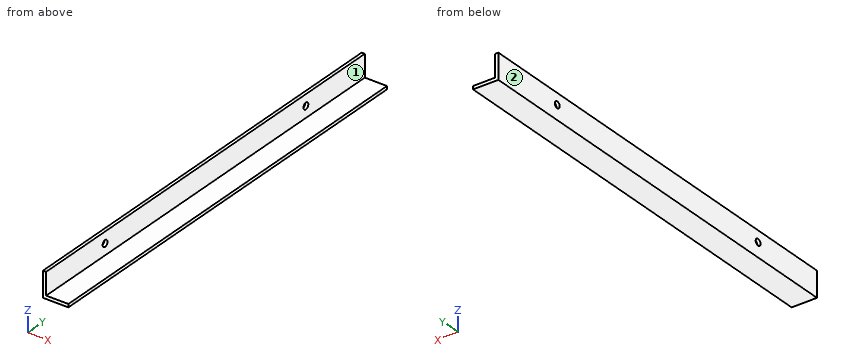
Autodesk Fusion 360 part; units mm, degrees
sketch "Sketch1" plane through (0, 0, 0) normal (0, 1, 0) x (1, 0, 0)
  line L0 (0, -25.4) -> (0, 0)
  line L1 (0, 0) -> (25.4, 0)
  line L2 (12.7, -12.7) -> (11.05, -11.05) construction
  line L3 (3.175, -25.4) -> (3.175, -3.175)
  line L4 (3.175, -3.175) -> (25.4, -3.175)
  line L5 (25.4, -3.175) -> (25.4, 0)
  line L6 (0, -25.4) -> (3.175, -25.4)
  dimension "d1" = 25.4
  dimension "d2" = 25.4
  dimension "d13" = 3.175
extrude "Extrude1" add sketch "Sketch1" along normal blind 215
hole "Hole3" at (3.175, 135.512, 14.2875) direction (-1, 0, 0) diameter 6.5 end through all
mirror "Mirror1" about plane through (0, 0, 0) normal (0, 1, 0) of bodies 1 merged
equation "d5 = ( 430 / 2 ) * 1 mm"
equation "d27 = ( 22.225 / 2 ) * 1 mm"
The model under review builds one solid part; all positions refer to its coordinate system, in mm. Face numbers are marked on the shaded views. A direction names the side the tool comes from. Round coordinates to 2 decimals unless told otherwise and drop trailing zeros. Write each loop counter-clockwise with the first axis right and the second up, starting at its lowest first coordinate (ties: lowest second). Pieces come first, ordered by that corner, then holes. Notation, with made-up numbers: M 10.25,80 L 57.25,80 A17 ccw 57.25,113 Z; hole C -21,41.5 d8. An arc over 180 degrees is marked long. Use CSV: the item, a comma, the result in double quotes. Start each with the question number.
(1) Tool access review of the marked faces 1 and 2: name each direction out of +Z, -Z, +X, -X, +Y, -Y from which nothing blocks a thin tool from reaching the whole face with its end or side.
(2) We need section A-A, the plane y = -1.5. State the section outline as (x, z) points (3 decimals), then the cut area to 3 significant figures.
(3) We need section B-B, the plane x = 7. State the section outline as (y, z) points (3 decimals), then the cut area to 3 significant figures.
(4) Clearance check with flat-ended pins moving along their axes: P1, Ø5, axis at y = -135.51, z = 14.29, coming from the -X side; P2, Ø6, axis at x = 7.5, y = 4.5, coming from the +Z side (3 decimals); P3, Ø8, axis at y = 9, z = 13, coming from the +X side (3 decimals). State where each tip first meets the part, or that it passes through.
(5) For line 1 along Z through (x, y) = (9.5, -92) (3 decimals), list the stretches that pass through material, from the lowest coordinate up.
(6) We need section C-C, the plane z = 21. State the section outline as (x, y) points (3 decimals), then the cut area to 3 significant figures.
Findings:
1,face 1,"+Z, +X, +Y, -Y"
1,face 2,"+Z, -Z, -X, +Y, -Y"
2,outline,"M 0,0 L 25.4,0 L 25.4,3.175 L 3.175,3.175 L 3.175,25.4 L 0,25.4 Z"
2,area,"151 mm^2"
3,outline,"M -215,0 L 215,0 L 215,3.175 L -215,3.175 Z"
3,area,"1,370 mm^2"
4,P1,"through"
4,P2,"z = 3.175"
4,P3,"x = 3.175"
5,line 1,"0 to 3.175"
6,outline,"M 0,-215 L 3.175,-215 L 3.175,215 L 0,215 Z"
6,area,"1,370 mm^2"
